```python
from build123d import *

# Parameters (mm, degrees)
F1_DEPTH      = 10
F1_DEPTH_BACK = 10
F3_DEPTH      = 8
F3_DEPTH_BACK = 8
F5_DEPTH      = 20.001
F6_R          = 3
F7_DEPTH      = 18.001
F8_W          = 12
F8_H          = 1.5
F9_DEPTH      = 10.001
F9_DEPTH_BACK = 10.001


with BuildPart() as f1:
    # F0 (on Top) → F1 (new body, two sides)
    with BuildSketch(Plane.XY) as f1_sk:
        with BuildLine():
            Line((12, 4), (9.1651513899, 4))
            ThreePointArc((9.1651513899, 4), (-10, 0), (9.1651513899, -4))
            Line((9.1651513899, -4), (12, -4))
            Line((12, -4), (12, 4))
        make_face()
    extrude(amount=F1_DEPTH)
    extrude(f1_sk.sketch, amount=-F1_DEPTH_BACK)

    # F2 (on Front) → F3 (join, two sides)
    with BuildSketch(Plane.XZ) as f3_sk:
        with BuildLine():
            Line((16, 5), (0, 5))
            Line((0, 5), (0, -5))
            Line((0, -5), (16, -5))
            ThreePointArc((16, -5), (21, 0), (16, 5))
        make_face()
    extrude(amount=F3_DEPTH)
    extrude(f3_sk.sketch, amount=-F3_DEPTH_BACK)

    # F4 (on face) → F5 (cut, through all)
    with BuildSketch(Plane.XY.offset(10)):
        with BuildLine():
            Line((10, 2), (7.7459666924, 2))
            ThreePointArc((7.7459666924, 2), (-8, 0), (7.7459666924, -2))
            Line((7.7459666924, -2), (10, -2))
            Line((10, -2), (10, 2))
        make_face()
    extrude(amount=-F5_DEPTH, mode=Mode.SUBTRACT)

    # F6 (on face) → F7 (cut, through all)
    with BuildSketch(Plane.XZ.offset(8)):
        with Locations((16, 0)):
            Circle(F6_R)
    extrude(amount=-F7_DEPTH, mode=Mode.SUBTRACT)

    # F8 (on Front) → F9 (cut, two sides)
    with BuildSketch(Plane.XZ) as f9_sk:
        with Locations((-6, 0)):
            Rectangle(F8_W, F8_H)
    extrude(amount=-F9_DEPTH, mode=Mode.SUBTRACT)
    extrude(f9_sk.sketch, amount=F9_DEPTH_BACK, mode=Mode.SUBTRACT)


solid = f1.part
```
Design review of the part built by this model. Coordinates are the model's own, in mm. A direction names the side the tool comes from. Coordinates: 2 decimals unless noted, no trailing zeros. Write each loop counter-clockwise with the first axis right and the second up, starting at its lowest first coordinate (ties: lowest second). Pieces come first, ordered by that corner, then holes.
1) Add section A-A (z = 0). Write out the cut boundary in (x, y), plus the area to 3 significant figures.
2) Add section C-C (z = 5.75). Write out the cut boundary in (x, y), plus the area to 3 significant figures.
3) Mouldability with a two-part tool opening along X and no side actions: class faces 1 (the flat face through (0, -9, 0)), 2 (the flat face through (7.5, 3.8, 10)), 3 (the flat face through (10, 0, 0)) as +X half, -X half, draft (parallel to the pull), parting line (faces both ways), or undercut.
4) Add section B-B (y = 0). Write out the cut boundary in (x, z).
5) To check wall thickness, follow L1, parallel to Z at x = 16, y = 0.25; L2, parallel to Y at x = 0, z = 2; L3, parallel to X at y = 0, z = 5.75. State the ranges of each line that lie inside material, in increasing order.
6) Insertion check: pin 1 (1.1 mm diameter, centred on x = 9, z = 3.5, fed in from -Y); pin 2 (1.1 mm diameter, centred on x = 9, z = -3.5, fed in from +Y); pin 3 (2 mm diameter, centred on y = -4, z = 5.5, fed in from -X). Each pin has a flat end and moves straight along its axis. Give the tip position at first contact, or say it passes through.
7) Add section D-D (y = 2.5). Write out the cut boundary in (x, z), plus the area to 3 significant figures.
8) Machinability: for faces 4 (the flat face through (9, -2, 0)), 5 (the flat face through (12, 0, 8)), 6 (the flat face through (11, 4, -7)), which of the approach directions +Z, -Z, +X, -X, +Y, -Y give a long, thin tool a straight path to every point of the face, cutting with its end or side? Answer none if there is none.
Check result:
1. outline: (0, -10) arc R10 ccw to (6, -8) - (13, -8) - (13, 8) - (6, 8) arc R10 ccw to (0, 10) - (0, 8) arc R8 cw to (7.75, 2) - (10, 2) - (10, -2) - (7.75, -2) arc R8 cw to (0, -8) - close; (19, -8) - (21, -8) - (21, 8) - (19, 8) - close
1. area: 147 mm2
2. outline: (9.17, -4) - (12, -4) - (12, 4) - (9.17, 4) arc R10 ccw (long way) to start; hole (7.75, -2) - (10, -2) - (10, 2) - (7.75, 2) arc R8 ccw (long way) to start
2. area: 123 mm2
3. face 1: -X half
3. face 2: draft
3. face 3: undercut
4. outline: (-10, -10) - (-8, -10) - (-8, -0.75) - (-10, -0.75) - close; (-10, 0.75) - (-8, 0.75) - (-8, 10) - (-10, 10) - close; (10, -10) - (12, -10) - (12, -5) - (16, -5) arc R5 ccw to (16, 5) - (12, 5) - (12, 10) - (10, 10) - close; hole circle Ø6 at (16, 0)
5. L1: z = -5 to -3, 3 to 5
5. L2: y = -10 to -8, 8 to 10
5. L3: x = -10 to -8, 10 to 12
6. pin 1: stops at y = -8
6. pin 2: stops at y = 8
6. pin 3: stops at x = -9.54
7. outline: (-9.68, -10) - (-7.6, -10) - (-7.6, -0.75) - (-9.68, -0.75) - close; (-9.68, 0.75) - (-7.6, 0.75) - (-7.6, 10) - (-9.68, 10) - close; (7.6, -10) - (12, -10) - (12, -5) - (16, -5) arc R5 ccw to (16, 5) - (12, 5) - (12, 10) - (7.6, 10) - close; hole circle Ø6 at (16, 0)
7. area: 178 mm2
8. face 4: +Z, -Z
8. face 5: +Z, +X, +Y, -Y
8. face 6: -Z, +X, +Y
